Build history of the part. All positions in model axes, mm. A direction names the side the tool comes from. Give positions to 0.01 mm unless a question says otherwise; leave off trailing zeros. Order: outer loops, then holes, each group sorted by start corner. A loop starts at its lowest first (then second) coordinate and runs counter-clockwise, first axis right, second up. Notation, with made-up numbers: (57, 20.25) - (92, 20.25) arc R18 cw to (92, 36.25) - close; hole circle Ø2 at (50.5, 55.5). An arc over 180 degrees is marked (long way). Use a Markdown table: item, result.
from build123d import *

# Parameters (mm, degrees)
F0_W     = 914.4
F0_H     = 2032
F1_DEPTH = 50.8
F2_W     = 152.4
F2_H     = 433.7214036722
F3_DEPTH = 15.24


with BuildPart() as f1:
    # F0 (on Front) → F1 (new body)
    with BuildSketch(Plane.XZ):
        with Locations((457.2, 1016)):
            Rectangle(F0_W, F0_H)
    extrude(amount=F1_DEPTH)

    # F2 (on face) → F3 (cut)
    with BuildSketch(Plane.XZ.offset(50.8)):
        Polygon((812.8, 1815.1392981639), (101.6, 1434.1392981639), (101.6, 1232.8607018361), (254, 1232.8607018361), (254, 1314.503558979), (812.8, 1613.8607018361), align=None)
        with Locations((177.8, 1016)):
            Rectangle(F2_W, F2_H)
        Polygon((812.8, 1930.4), (101.6, 1930.4), (101.6, 1549.4), align=None)
        Polygon((254, 799.1392981639), (101.6, 799.1392981639), (101.6, 597.8607018361), (812.8, 216.8607018361), (812.8, 418.1392981639), (254, 717.496441021), align=None)
        Polygon((101.6, 101.6), (812.8, 101.6), (101.6, 482.6), align=None)
    extrude(amount=-F3_DEPTH, mode=Mode.SUBTRACT)


solid = f1.part
1) Wall check: line 1 (Z direction, x = 298, y = -46.5); line 2 (Z direction, x = 683, y = -38); line 3 (Y direction, x = 544, z = 1891). Give the ranges that are in metal, low to high. Write a range as from..to.
Computed:
| item | result |
|---|---|
| line 1 | z = 0..101.6, 377.39..492.65, 693.93..1338.07, 1539.35..1654.61, 1930.4..2032 |
| line 2 | z = 0..101.6, 171.14..286.4, 487.68..1544.32, 1745.6..1860.86, 1930.4..2032 |
| line 3 | y = -35.56..0 |
2) Slice it at D-D (x = 338). Write the cut outline in (y, z).
Computed:
| item | result |
|---|---|
| outline | (-50.8, 0) - (0, 0) - (0, 2032) - (-50.8, 2032) - (-50.8, 1930.4) - (-35.56, 1930.4) - (-35.56, 1676.04) - (-50.8, 1676.04) - (-50.8, 1560.78) - (-35.56, 1560.78) - (-35.56, 1359.5) - (-50.8, 1359.5) - (-50.8, 672.5) - (-35.56, 672.5) - (-35.56, 471.22) - (-50.8, 471.22) - (-50.8, 355.96) - (-35.56, 355.96) - (-35.56, 101.6) - (-50.8, 101.6) - close |
3) Pin check, flat tip, straight feed: P1, Ø10, axis at x = 499.5, y = -12.5, coming from the -Z side. Stop position of the tip, or through.
Computed:
| item | result |
|---|---|
| P1 | stops at z = 0 |
4) Tool access for faces 1 (the flat face through (451, -50.8, 1030)), 2 (the flat face through (294, -35.56, 210)): list every direction of +Z, -Z, +X, -X, +Y, -Y with a clear straight run to the whole face (end or side of a thin tool).
Computed:
| item | result |
|---|---|
| face 1 | +Z, -Z, +X, -X, -Y |
| face 2 | -Y |
5) Slice it at B-B (x = 681). Write the cut outline in (y, z).
Computed:
| item | result |
|---|---|
| outline | (-50.8, 0) - (0, 0) - (0, 2032) - (-50.8, 2032) - (-50.8, 1930.4) - (-35.56, 1930.4) - (-35.56, 1859.79) - (-50.8, 1859.79) - (-50.8, 1744.53) - (-35.56, 1744.53) - (-35.56, 1543.25) - (-50.8, 1543.25) - (-50.8, 488.75) - (-35.56, 488.75) - (-35.56, 287.47) - (-50.8, 287.47) - (-50.8, 172.21) - (-35.56, 172.21) - (-35.56, 101.6) - (-50.8, 101.6) - close |
6) Two-plate mould, pull along X, no slides. Class faces 3 (the flat face through (0, -25, 1002)), 4 (the flat face through (451, 0, 1030)), 5 (the flat face through (245, -35.56, 961)): +X half, -X half, draft (parallel to the pull), parting line (faces both ways), or undercut.
Computed:
| item | result |
|---|---|
| face 3 | -X half |
| face 4 | draft |
| face 5 | undercut |
7) Slice it at A-A (z = 1248). Write the cut outline in (x, y), and give its area (3 significant figures).
Computed:
| item | result |
|---|---|
| outline | (0, -50.8) - (101.6, -50.8) - (101.6, -35.56) - (254, -35.56) - (254, -50.8) - (914.4, -50.8) - (914.4, 0) - (0, 0) - close |
| area | 44,100 mm² |
8) Slice it at C-C (z = 580). Write the cut outline in (x, y).
Computed:
| item | result |
|---|---|
| outline | (0, -50.8) - (134.94, -50.8) - (134.94, -35.56) - (510.66, -35.56) - (510.66, -50.8) - (914.4, -50.8) - (914.4, 0) - (0, 0) - close |
